```python
from build123d import *

# Parameters (mm, degrees)
F0_R     = 18
F1_DEPTH = 64
F2_R     = 7
F3_DEPTH = 25
F4_DEPTH = 4
F5_SIZE2 = 1
F5_SIZE  = 1
F6_SIZE2 = 2
F6_SIZE  = 2
F7_R     = 10


with BuildPart() as f1:
    # F0 (on Front) → F1 (new body)
    with BuildSketch(Plane.XZ):
        with BuildLine():
            ThreePointArc((0, -30), (21.213203, -21.213203), (30, 0))
            ThreePointArc((30, 0), (-21.213203, 21.213203), (0, -30))
        make_face()
        Circle(F0_R, mode=Mode.SUBTRACT)
        with BuildLine():
            Line((30, -18), (30, 0))
            ThreePointArc((30, 0), (21.213203, -21.213203), (0, -30))
            Line((0, -30), (40, -30))
            Line((40, -30), (40, -34))
            Line((40, -34), (52, -34))
            Line((52, -34), (80, -34))
            Line((80, -34), (92, -34))
            Line((92, -34), (92, -18))
            Line((92, -18), (30, -18))
        make_face()
    extrude(amount=F1_DEPTH)

    # F2 (on face) → F3 (cut)
    with BuildSketch(Plane(origin=(0, 0, -34), x_dir=(1, 0, 0), z_dir=(0, 0, -1))):
        with BuildLine():
            ThreePointArc((52, 64), (55.662129, 63.427546), (58.974858, 61.764802))
            Line((58.974858, 61.764802), (86.974858, 41.764802))
            ThreePointArc((86.974858, 41.764802), (90.670012, 37.490979), (92, 32))
            Line((92, 32), (92, 64))
            Line((92, 64), (52, 64))
        make_face()
        with BuildLine():
            Line((92, 0), (92, 32))
            ThreePointArc((92, 32), (90.670012, 26.509021), (86.974858, 22.235198))
            Line((86.974858, 22.235198), (58.974858, 2.235198))
            ThreePointArc((58.974858, 2.235198), (55.662129, 0.572454), (52, 0))
            Line((52, 0), (92, 0))
        make_face()
        with Locations((52, 52)):
            Circle(F2_R)
        with Locations((52, 12)):
            Circle(F2_R)
        with Locations((80, 32)):
            Circle(F2_R)
    extrude(amount=-F3_DEPTH, mode=Mode.SUBTRACT)

    # F2 (on face) → F4 (cut)
    with BuildSketch(Plane(origin=(0, 0, -34), x_dir=(1, 0, 0), z_dir=(0, 0, -1))):
        with BuildLine():
            ThreePointArc((40, 52), (43.514719, 60.485281), (52, 64))
            Line((52, 64), (40, 64))
            Line((40, 64), (40, 52))
        make_face()
        with BuildLine():
            ThreePointArc((52, 0), (43.514719, 3.514719), (40, 12))
            Line((40, 12), (40, 0))
            Line((40, 0), (52, 0))
        make_face()
    extrude(amount=-F4_DEPTH, mode=Mode.SUBTRACT)

    # F5
    f5_edges = [f1.edges().sort_by_distance(p)[0] for p in [
        (45, -12, -18),
        (73, -32, -18),
        (45, -52, -18),
        (45, -52, -34),
        (73, -32, -34),
        (45, -12, -34),
    ]]
    chamfer(f5_edges, length=F5_SIZE, length2=F5_SIZE2)

    # F6
    f6_edges = [f1.edges().sort_by_distance(p)[0] for p in [
        (-18, 0, 0),
        (-18, -64, 0),
    ]]
    chamfer(f6_edges, length=F6_SIZE, length2=F6_SIZE2)

    # F7
    f7_edges = [f1.edges().sort_by_distance(p)[0] for p in [
        (30, -32, -18),
    ]]
    fillet(f7_edges, radius=F7_R)


solid = f1.part
```
For this review, take the finished solid that the model builds, in its own axes (mm). A direction names the side the tool comes from. Coordinates: 2 decimals unless noted, no trailing zeros. Order: outer loops, then holes, each group sorted by start corner. A loop starts at its lowest first (then second) coordinate and runs counter-clockwise, first axis right, second up. Notation, with made-up numbers: (-34.75, 37.5) - (-27.75, 37.5) arc R25 cw to (-27.75, 72.5) - close; hole circle Ø7 at (-4, 44). An arc over 180 degrees is marked (long way). Answer as a JSON object with one key per item and string values. Group by question number.
1. Clearance check with flat-ended pins moving along their axes: P1, Ø12, axis at y = -22.5, z = -9.5, coming from the -X side; P2, Ø10, axis at y = -51, z = 12, coming from the +X side; P3, Ø6, axis at x = -15, y = -14, coming from the -Z side; P4, Ø12, axis at x = 10.5, z = 12.5, coming from the -Y side. State where each tip first meets the part, or that it passes through.
2. The part is to be moulded in two halves that separate along Z. For faces 4 (the flat face through (30, -32, -4)), 5 (the cylindrical face through (33.01, -32.45, -15.15)), 6 (the cylindrical face through (-2.343, -31.58, 17.847)), say which applies: pulls with the +Z half, pulls with the -Z half, needs draft (parallel to the pull), parting line crosses it, or undercut.
3. We need section A-A on x = 80. State the section outline as (y, z) points, then the cut area to 3 significant figures.
4. For probe 1 along Y at (x, z) = (52, -26); probe 2 along Z at (x, y) = (46, -21.5); probe 3 along X at (y, z) = (-13.5, -1), list the stretches that pass through material, from the lowest coordinate up.
5. For faces 1 (the flat face through (40, -32, -32)), 2 (the flat face through (60, -32, -34)), 3 (the flat face through (61, -32, -18)), list the 3-axis set-ups (+Z, -Z, +X, -X, +Y, -Y) from which the entire face can be reached by the end or side of a thin tool; tool diameter is ignored.
6. We need section B-B on x = 34. State the section outline as (y, z) points, then the cut area to 3 significant figures.
7. We need section C-C on y = -27. Give the number of separate pieces and of enclosed holes in the cut face, then the cut area to 3 significant figures.
Final values:
{
 "1": {"P1": "x = -29.8", "P2": "x = 29.17", "P3": "z = -27.5", "P4": "y = -64"},
 "2": {"face 4": "needs draft", "face 5": "pulls with the +Z half", "face 6": "undercut"},
 "3": {"outline": "(-46.75, -34) - (-40, -34) - (-39, -33) - (-39, -19) - (-40, -18) - (-46.75, -18) - close; (-25, -33) - (-24, -34) - (-17.25, -34) - (-17.25, -18) - (-24, -18) - (-25, -19) - close", "area": "246 mm²"},
 "4": {"probe 1": "-64 to -59, -45 to -19, -5 to 0", "probe 2": "-34 to -18", "probe 3": "-29.98 to -17.97, 17.97 to 30"},
 "5": {"face 1": "-Z, -X, +Y, -Y", "face 2": "-Z, +X, -X, +Y, -Y", "face 3": "+Z, +X, +Y, -Y"},
 "6": {"outline": "(-64, -30) - (0, -30) - (0, -16) - (-64, -16) - close", "area": "896 mm²"},
 "7": {"separate pieces": "2", "enclosed holes": "1", "area": "2,800 mm²"}
}
